from build123d import *

# Parameters (mm, degrees)
F1_DEPTH = 7
F2_R     = 0.99999


# Not quite as in the source:
# - a fillet or chamfer is up to 0.001 mm smaller than in the source, because OpenCascade refuses the exact size


with BuildPart() as f1:
    # F0 (on Top) → F1 (new body)
    with BuildSketch(Plane.XY):
        Polygon((4.1, 1.5), (0, 1.5), (-4.1, 1.5), (-4.1, 12.5), (-6.1, 12.5), (-6.1, -12.5), (-3.5, -12.5), (-3.5, -1.5), (0, -1.5), (3.5, -1.5), (3.5, -12.5), (6.1, -12.5), (6.1, 12.5), (4.1, 12.5), align=None)
    extrude(amount=F1_DEPTH)

    # F2 (radius 1 in the source; OpenCascade refuses exactly that, so slightly less here)
    f2_edges = [f1.edges().sort_by_distance(p)[0] for p in [
        (3.5, -12.5, 3.5),
        (6.1, -12.5, 3.5),
        (-3.5, -12.5, 3.5),
        (-6.1, -12.5, 3.5),
        (6.1, 12.5, 3.5),
        (4.1, 12.5, 3.5),
        (-4.1, 12.5, 3.5),
        (-6.1, 12.5, 3.5),
    ]]
    fillet(f2_edges, radius=F2_R)


solid = f1.part
The model under review builds one solid part; all positions refer to its coordinate system, in mm. A direction names the side the tool comes from. Round coordinates to 2 decimals unless told otherwise and drop trailing zeros. Write each loop counter-clockwise with the first axis right and the second up, starting at its lowest first coordinate (ties: lowest second). Pieces come first, ordered by that corner, then holes. Notation, with made-up numbers: (85.25, 53) -> (143.25, 53) arc R9 ccw to (143.25, 59) -> close; hole circle Ø11 at (52, -21.5). An arc over 180 degrees is marked (long way). Answer as a JSON object with one key per item and string values.
1. To check wall thickness, follow line 1 along X through (y, z) = (-7.75, 3.5); line 2 along X through (y, z) = (4, 3.5); line 3 along Y through (x, z) = (-3, 3.5). State the ranges of each line that lie inside material, in increasing order.
Results found:
{"line 1": "x = -6.1 to -3.5, 3.5 to 6.1", "line 2": "x = -6.1 to -4.1, 4.1 to 6.1", "line 3": "y = -1.5 to 1.5"}
2. We need section A-A on y = 2. State the section outline as (x, z) points.
Results found:
{"outline": "(-6.1, 0) -> (-4.1, 0) -> (-4.1, 7) -> (-6.1, 7) -> close; (4.1, 0) -> (6.1, 0) -> (6.1, 7) -> (4.1, 7) -> close"}
3. We need section D-D on x = -0.75. State the section outline as (y, z) points, and give its area (3 significant figures).
Results found:
{"outline": "(-1.5, 0) -> (1.5, 0) -> (1.5, 7) -> (-1.5, 7) -> close", "area": "21.0 mm^2"}
4. Clearance check with a flat-ended pin moving along its axis: pin 1 (3.5 mm diameter, centred on x = 1, z = 2, fed in from +Y). State where the tip first meets the part, or that it passes through.
Results found:
{"pin 1": "stops at y = 1.5"}
5. The part is to be moulded in two halves that separate along X. For faces 4 (the face through (-5.815, -12.199, 3.549)), 5 (the face through (0, -1.5, 3)), 6 (the face through (5.799, -12.215, 3.549)), say which applies: pulls with the +X half, pulls with the -X half, needs draft (parallel to the pull), parting line crosses it, or undercut.
Results found:
{"face 4": "pulls with the -X half", "face 5": "undercut", "face 6": "pulls with the +X half"}
6. Machinability: for faces 1 (the face through (-3.5, -7, 3)), 2 (the face through (6.1, 0, 3)), 3 (the face through (0, 1.5, 3)), which of the approach directions +Z, -Z, +X, -X, +Y, -Y give a long, thin tool a straight path to every point of the face, cutting with its end or side? Answer none if there is none.
Results found:
{"face 1": "+Z, -Z, -Y", "face 2": "+Z, -Z, +X, +Y, -Y", "face 3": "+Z, -Z, +Y"}
7. We need section C-C on y = -3. State the section outline as (x, z) points, and give its area (3 significant figures).
Results found:
{"outline": "(-6.1, 0) -> (-3.5, 0) -> (-3.5, 7) -> (-6.1, 7) -> close; (3.5, 0) -> (6.1, 0) -> (6.1, 7) -> (3.5, 7) -> close", "area": "36.4 mm^2"}
